from build123d import *

# Parameters (mm, degrees)
CROQUIS13_R                = 5
CROQUIS13_R_2              = 6
SALIENTE_EXTRUIR1_DEPTH    = 4.765
REDONDEO2_R                = 0.3
REDONDEO3_R                = 80
REDONDEO4_R                = 15
CORTAR_EXTRUIR2_REACH      = 170.937
CROQUIS18_R                = 3.125
CORTAR_EXTRUIR3_DEPTH      = 169.735607463
CORTAR_EXTRUIR3_DEPTH_BACK = 169.735607463
REDONDEO5_R                = 3
CORTAR_EXTRUIR4_DEPTH      = 169.735607463
CORTAR_EXTRUIR4_DEPTH_BACK = 169.735607463
CROQUIS21_R                = 7.94


with BuildPart() as part:
    # Croquis13 → Saliente-Extruir1 (new, symmetric)
    with BuildSketch(Plane(origin=(0, 0, 0), x_dir=(0, 0, -1), z_dir=(1, 0, 0))):
        with BuildLine():
            Line((102.163414857, -4.327209349), (81.574356475, 9.853435029))
            ThreePointArc((81.574356475, 9.853435029), (77.521218134, 11.823084958), (73.065969849, 12.5))
            Line((73.065969849, 12.5), (-16.81645687, 12.5))
            ThreePointArc((-16.81645687, 12.5), (-20.351990776, 11.035533906), (-21.81645687, 7.5))
            Line((-21.81645687, 7.5), (-21.81645687, -8.626101457))
            ThreePointArc((-21.81645687, -8.626101457), (-20.351990776, -12.161635363), (-16.81645687, -13.626101457))
            Line((-16.81645687, -13.626101457), (43.18354313, -13.626101457))
            ThreePointArc((43.18354313, -13.626101457), (76.306099966, -44.847644025), (92.158871945, -87.515877082))
            ThreePointArc((92.158871945, -87.515877082), (113.995550437, -104.900195438), (131.945619804, -83.526144302))
            ThreePointArc((131.945619804, -83.526144302), (122.754645176, -41.783183661), (102.163414857, -4.327209349))
        make_face()
        with Locations((27, 0)):
            Circle(CROQUIS13_R, mode=Mode.SUBTRACT)
        Circle(CROQUIS13_R, mode=Mode.SUBTRACT)
        with Locations((112, -85)):
            Circle(CROQUIS13_R_2, mode=Mode.SUBTRACT)
    extrude(amount=SALIENTE_EXTRUIR1_DEPTH, both=True)

    # Croquis15 → Cortar-Revolución2 (revolve, cut)
    with BuildSketch(Plane(origin=(0, -85, 0), x_dir=(1, 0, 0), z_dir=(0, 1, 0)), mode=Mode.PRIVATE) as cortar_revoluci_n2_sk:
        Polygon((4.765, 106.01), (4.765, 100), (3.765, 100), (-2.245, 106.01), align=None)
    revolve(cortar_revoluci_n2_sk.sketch.rotate(Axis((4.765, -85, -112), (-1, 0, 0)), 180), axis=Axis((4.765, -85, -112), (-1, 0, 0)), mode=Mode.SUBTRACT)

    # Redondeo2
    redondeo2_edges = [part.edges().sort_by_distance(p)[0] for p in [
        (4.765, -85, -100),
    ]]
    fillet(redondeo2_edges, radius=REDONDEO2_R)

    # Redondeo3
    redondeo3_edges = [part.edges().sort_by_distance(p)[0] for p in [
        (0, -13.626101457, -43.18354313),
    ]]
    fillet(redondeo3_edges, radius=REDONDEO3_R)

    # Redondeo4
    redondeo4_edges = [part.edges().sort_by_distance(p)[0] for p in [
        (0, -4.327209349, -102.163414857),
    ]]
    fillet(redondeo4_edges, radius=REDONDEO4_R)

    # Croquis18 → Cortar-Extruir2 (cut, up to next)
    with BuildSketch(Plane.ZY.offset(4.765), mode=Mode.PRIVATE) as cortar_extruir2_sk1:
        with Locations((-97.175215853, -60)):
            Circle(CROQUIS18_R)
    cortar_extruir2_tool1 = extrude(cortar_extruir2_sk1.sketch, amount=-CORTAR_EXTRUIR2_REACH, mode=Mode.PRIVATE) & part.part
    # Croquis18 → Cortar-Extruir2 (cut, up to next)
    with BuildSketch(Plane.ZY.offset(4.765), mode=Mode.PRIVATE) as cortar_extruir2_sk2:
        with Locations((-116.837549653, -56.340405824)):
            Circle(CROQUIS18_R)
    cortar_extruir2_tool2 = extrude(cortar_extruir2_sk2.sketch, amount=-CORTAR_EXTRUIR2_REACH, mode=Mode.PRIVATE) & part.part
    # Croquis18 → Cortar-Extruir2 (cut, up to next)
    with BuildSketch(Plane.ZY.offset(4.765), mode=Mode.PRIVATE) as cortar_extruir2_sk3:
        with Locations((-106.681694763, -56.425713405)):
            Circle(CROQUIS18_R)
    cortar_extruir2_tool3 = extrude(cortar_extruir2_sk3.sketch, amount=-CORTAR_EXTRUIR2_REACH, mode=Mode.PRIVATE) & part.part
    add(cortar_extruir2_tool1.solids().sort_by_distance((-4.765, -60, -97.175216))[0], mode=Mode.SUBTRACT)
    add(cortar_extruir2_tool2.solids().sort_by_distance((-4.765, -56.340406, -116.83755))[0], mode=Mode.SUBTRACT)
    add(cortar_extruir2_tool3.solids().sort_by_distance((-4.765, -56.425713, -106.681695))[0], mode=Mode.SUBTRACT)

    # Croquis20 → Cortar-Extruir3 (cut, two sides: drawn at the far end of the back side and taken through both)
    with BuildSketch(Plane(origin=(0, 0, 0), x_dir=(0, 0, -1), z_dir=(1, 0, 0)).offset(-CORTAR_EXTRUIR3_DEPTH_BACK)):
        with BuildLine():
            Line((-21.81645687, 7.5), (-21.81645687, -8.626101457))
            ThreePointArc((-21.81645687, -8.626101457), (-20.351990776, -12.161635363), (-16.81645687, -13.626101457))
            Line((-16.81645687, -13.626101457), (-9.81645687, -13.626101457))
            Line((-9.81645687, -13.626101457), (-9.81645687, 12.5))
            Line((-9.81645687, 12.5), (-16.81645687, 12.5))
            ThreePointArc((-16.81645687, 12.5), (-20.351990776, 11.035533906), (-21.81645687, 7.5))
        make_face()
    extrude(amount=CORTAR_EXTRUIR3_DEPTH + CORTAR_EXTRUIR3_DEPTH_BACK, mode=Mode.SUBTRACT)

    # Redondeo5
    redondeo5_edges = [part.edges().sort_by_distance(p)[0] for p in [
        (0, 12.5, 9.81645687),
        (0, -13.626101457, 9.81645687),
    ]]
    fillet(redondeo5_edges, radius=REDONDEO5_R)

    # Croquis21 → Cortar-Extruir4 (cut, two sides: drawn at the far end of the back side and taken through both)
    with BuildSketch(Plane(origin=(0, 0, 0), x_dir=(0, 0, -1), z_dir=(1, 0, 0)).offset(-CORTAR_EXTRUIR4_DEPTH_BACK)):
        Circle(CROQUIS21_R)
    extrude(amount=CORTAR_EXTRUIR4_DEPTH + CORTAR_EXTRUIR4_DEPTH_BACK, mode=Mode.SUBTRACT)


solid = part.part
The listing builds one solid part. Answer for the finished solid, in the listing's coordinates (mm). A direction names the side the tool comes from. Give positions to 0.01 mm unless a question says otherwise; leave off trailing zeros. Write each loop counter-clockwise with the first axis right and the second up, starting at its lowest first coordinate (ties: lowest second). Pieces come first, ordered by that corner, then holes. Notation, with made-up numbers: (29.25, 77.25) -> (70.25, 77.25) arc R15 cw to (70.25, 97.25) -> close; hole circle Ø6 at (-20.5, 0). An arc over 180 degrees is marked (long way). Use a Markdown table: item, result.
(1) Section A-A, the plane z = 0 is taken. Determine the outline of the cut face in (x, y) (3 decimals).
Return value:
| item | result |
|---|---|
| outline | (-4.765, -13.626) -> (4.765, -13.626) -> (4.765, -7.94) -> (-4.765, -7.94) -> close; (-4.765, 7.94) -> (4.765, 7.94) -> (4.765, 12.5) -> (-4.765, 12.5) -> close |
(2) Section D-D, the plane z = -79 is taken. Determine the outline of the cut face in (x, y) (3 decimals).
Return value:
| item | result |
|---|---|
| outline | (-4.765, -50.099) -> (4.765, -50.099) -> (4.765, 11.276) -> (-4.765, 11.276) -> close |
(3) Determine the mould class of faces 1 (the cylindrical face through (0.067, -12.771, 8.914)), 2 (the cylindrical face through (0.067, -43.567, -123.412)), 3 (the conical face through (-1.944, -78.858, -110.636)), 4 (the cylindrical face through (4.11, -85.53, -100.01)) for opening direction Y: released by +Y, released by -Y, zero draft, split by the parting line, or undercut.
Return value:
| item | result |
|---|---|
| face 1 | released by -Y |
| face 2 | released by +Y |
| face 3 | undercut |
| face 4 | undercut |
(4) Find the intervals of material crossed by probe 1 along Z at (x, y) = (-3, -54.5); probe 2 along Y at (x, z) = (-0.25, -107.5); probe 3 along Y at (x, z) = (-2, -2.5), in increasing order. Write a range as from..to.
Return value:
| item | result |
|---|---|
| probe 1 | -126.9..-119.36, -114.31..-109.14, -104.22..-81.66 |
| probe 2 | -104.49..-91.6, -78.4..-59.44, -53.41..-11.89 |
| probe 3 | -13.63..-7.54, 7.54..12.5 |
(5) Section B-B, the plane y = 0 is taken. Determine the outline of the cut face in (x, z) (3 decimals), then the cut area to 3 significant figures.
Return value:
| item | result |
|---|---|
| outline | (-4.765, -95.881) -> (4.765, -95.881) -> (4.765, -32) -> (-4.765, -32) -> close; (-4.765, -22) -> (4.765, -22) -> (4.765, -7.94) -> (-4.765, -7.94) -> close; (-4.765, 7.94) -> (4.765, 7.94) -> (4.765, 9.816) -> (-4.765, 9.816) -> close |
| area | 761 mm2 |
(6) For faces 5 (the cylindrical face through (-0.07, -57.89, -99.48)), 6 (the flat face through (0, -13.626, -2)), determine the directions among +Z, -Z, +X, -X, +Y, -Y from which every point of the face is accessible in a straight line to the end or side of a thin tool.
Return value:
| item | result |
|---|---|
| face 5 | +X, -X |
| face 6 | +Z, +X, -X, -Y |
(7) Flat-ended cylindrical pins translate along their axes: P1, Ø3, axis at x = 3.5, z = -99, coming from the -Y side; P2, Ø5, axis at x = -2.5, z = -2.5, coming from the -Y side; P3, Ø5, axis at y = -56.34, z = -116.84, coming from the +X side; P4, Ø3, axis at x = 2, z = -77.5, coming from the +Y side. Find the tip coordinate at first contact, or state that the pin passes through.
Return value:
| item | result |
|---|---|
| P1 | y = -101.36 |
| P2 | y = -13.63 |
| P3 | through |
| P4 | y = 12.21 |
(8) Section C-C, the plane z = -112 is taken. Determine the outline of the cut face in (x, y) (3 decimals), then the cut area to 3 significant figures.
Return value:
| item | result |
|---|---|
| outline | (-4.765, -105) -> (4.765, -105) -> (4.765, -97.3) arc R0.3 ccw to (4.465, -97) -> (3.765, -97) -> (-2.235, -91) -> (-4.765, -91) -> close; (-4.765, -79) -> (-2.235, -79) -> (3.765, -73) -> (4.465, -73) arc R0.3 ccw to (4.765, -72.7) -> (4.765, -19.136) -> (-4.765, -19.136) -> close |
| area | 656 mm2 |
